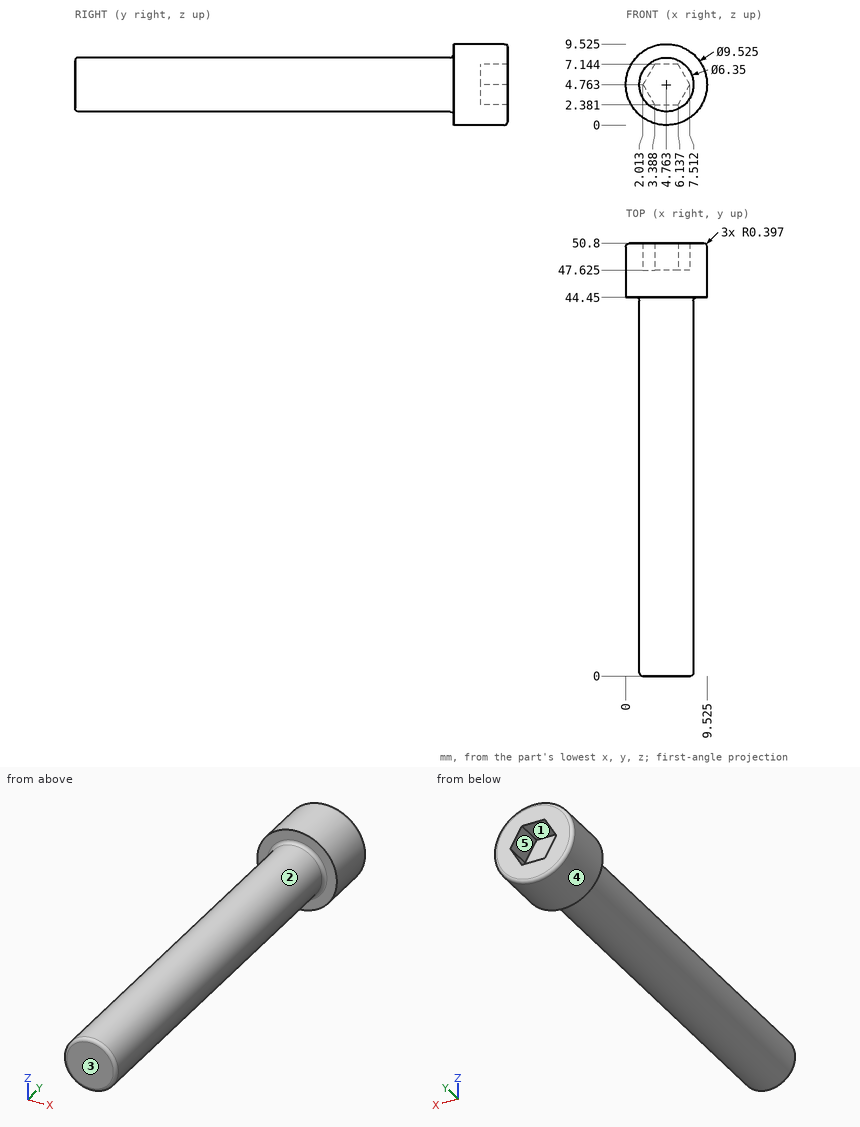
Job drawing, mm, ordinate dimensions from the low corner. One solid piece. A direction names the side the tool comes from. Round coordinates to 2 decimals unless told otherwise and drop trailing zeros.
(1) Which spindle directions (+Z, -Z, +X, -X, +Y, -Y) get a long thin tool onto all of the face, cutting with end or side? Do the marked faces 4 and 5. Say none if no direction does.
(2) Drop flat-ended pins along their axis: pin 1 (1.5 mm diameter, centred on x = 7.5, y = 35.5, fed in from +Z); pin 2 (3 mm diameter, centred on y = 23.5, z = 1.5, fed in from -X); pin 3 (1.5 mm diameter, centred on x = 5.5, y = 33, fed in from -Z). Give the stop position or say it passes through.
(3) Wall check: line 1 along X through (y, z) = (42, 5); line 2 along Y through (x, z) = (8.75, 4.5); line 3 along Y through (x, z) = (5.75, 5) (1 decimal). Give the ranges that are in metal, low to high.
(4) Two-plate mould, pull along Z, no slides. Class the marked faces 1, 2 and 3: +Z half, -Z half, draft (parallel to the pull), parting line (faces both ways), or undercut.
Findings below:
1. face 4: +Y, -Y
1. face 5: +Y
2. pin 1: stops at z = 7.24
2. pin 2: stops at x = 2.12
2. pin 3: stops at z = 1.59
3. line 1: x = 1.6 to 7.93
3. line 2: y = 44.45 to 50.8
3. line 3: y = 0 to 47.6
4. face 1: undercut
4. face 2: parting line
4. face 3: draft
